Source: CAD feature listing. Evaluate the final solid. Frame: model axes, mm. A direction names the side the tool comes from. Give positions to 0.01 mm unless a question says otherwise; leave off trailing zeros. Loops run counter-clockwise (first coordinate to the right, second up) from the corner with the lowest first, then second, coordinate; pieces in that order, holes last. Notation, with made-up numbers: (74.5, 15) -> (127.5, 15) arc R21 ccw to (127.5, 47) -> close; hole circle Ø2 at (17, 20.25). An arc over 180 degrees is marked (long way). Return JSON: item names as keys, results as strings. Group by question number.
```python
from build123d import *
from build123d.topology import SkipClean

# Parameters (mm, degrees)
SKETCH7_R                  = 38.1
SKETCH7_R_2                = 18.1229
BOSS_EXTRUDE3_DEPTH        = 9.525
CUT_EXTRUDE4_REACH         = 1065.597
CUT_EXTRUDE4_END_RADIUS    = 31.75
CIRPATTERN1_COUNT          = 6
SKETCH19_R                 = 38.1
BOSS_EXTRUDE4_DEPTH        = 15.875
F_10_32_TAPPED_HOLE1_D     = 4.0386
F_10_32_TAPPED_HOLE1_DEPTH = 12.7
F_10_32_TAPPED_HOLE1_TIP   = 1.213317848


with BuildPart() as part:
    # Sketch1 → Revolve1 (revolve)
    with BuildSketch(Plane.XY, mode=Mode.PRIVATE) as revolve1_sk:
        Polygon((104.775, 1038.225), (104.775, 1044.575), (114.3, 1044.575), (114.3, 1054.1), (120.65, 1054.1), (120.65, 1044.575), (133.582417551, 1044.575), (133.582417551, 1038.225), align=None)
    revolve(revolve1_sk.sketch.rotate(Axis((184.382417551, 1006.475, 0), (-1, 0, 0)), 90), axis=Axis((184.382417551, 1006.475, 0), (-1, 0, 0)))

    # Sketch7 → Boss-Extrude3 (add)
    with BuildSketch(Plane(origin=(133.582417551, 0, 0), x_dir=(0, 0, -1), z_dir=(1, 0, 0))):
        with Locations((0, 1006.475)):
            Circle(SKETCH7_R)
        with Locations((0, 1006.475)):
            Circle(SKETCH7_R_2, mode=Mode.SUBTRACT)
    extrude(amount=-BOSS_EXTRUDE3_DEPTH)

    # Cut-Extrude4: up to this cylinder (the profile starts inside it)
    cut_extrude4_end = Plane(origin=(128.8199175, 1006.475, 0), z_dir=(1, 0, 0)) * Cylinder(CUT_EXTRUDE4_END_RADIUS, 2204.478263, mode=Mode.PRIVATE)
    # Sketch8 → Cut-Extrude4 (cut, up to the surface)
    with BuildSketch(Plane.XY, mode=Mode.PRIVATE) as cut_extrude4_sk1:
        Polygon((133.582417551, 1000.125), (133.582417551, 1012.825), (132.471311524, 1000.125), align=None)
    cut_extrude4_tool1 = extrude(cut_extrude4_sk1.sketch, amount=-CUT_EXTRUDE4_REACH, mode=Mode.PRIVATE) & cut_extrude4_end
    # Sketch8 → Cut-Extrude4 (cut, up to the surface)
    with BuildSketch(Plane.XY, mode=Mode.PRIVATE) as cut_extrude4_sk2:
        Polygon((124.057417551, 1012.825), (124.057417551, 1000.125), (125.168523578, 1012.825), align=None)
    cut_extrude4_tool2 = extrude(cut_extrude4_sk2.sketch, amount=-CUT_EXTRUDE4_REACH, mode=Mode.PRIVATE) & cut_extrude4_end
    cut_extrude4 = cut_extrude4_tool1.solids().sort_by_distance((133.212049, 1004.358333, 0))[0] + cut_extrude4_tool2.solids().sort_by_distance((124.427786, 1008.591667, 0))[0]
    add(cut_extrude4, mode=Mode.SUBTRACT)

    # Sketch18 → #10-24 Tapped Hole2 (revolve, cut)
    with BuildSketch(Plane(origin=(133.031084587, 1006.523235384, -22.225), x_dir=(0.08715574274765736, 0.9961946980917457, 0), z_dir=(0, 0, 1))):
        Polygon((0, 0), (0, 16.126824014), (1.89865, 14.986), (1.89865, 0), align=None)
    f_10_24_tapped_hole2 = revolve(axis=Axis((139.35692092, 1005.969796418, -22.225), (-0.9961946980917457, 0.08715574274765729, 0)), mode=Mode.SUBTRACT)

    # CirPattern1: Cut-Extrude4, #10-24 Tapped Hole2 ×6 about axis
    with SkipClean():  # the faces are left unmerged after this step: merging them gives an invalid solid
        cirpattern1_axis = Axis((0, 1006.475, 0), (1, 0, 0))
        add([cut_extrude4.rotate(cirpattern1_axis, i * 360 / CIRPATTERN1_COUNT) for i in range(1, CIRPATTERN1_COUNT)], mode=Mode.SUBTRACT)
        add([f_10_24_tapped_hole2.rotate(cirpattern1_axis, i * 360 / CIRPATTERN1_COUNT) for i in range(1, CIRPATTERN1_COUNT)], mode=Mode.SUBTRACT)
    add(part.part.scale(1), mode=Mode.REPLACE)  # the faces are merged on a copy

    # Sketch19 → Boss-Extrude4 (add)
    with SkipClean():  # the faces are left unmerged after this step: merging them gives an invalid solid
        with BuildSketch(Plane.ZY.offset(-120.65)):
            with BuildLine():
                Line((-47.625, 1006.475), (-47.625, 1057.275))
                Line((-47.625, 1057.275), (47.625, 1057.275))
                Line((47.625, 1057.275), (47.625, 1006.475))
                ThreePointArc((47.625, 1006.475), (0, 958.85), (-47.625, 1006.475))
            make_face()
            with Locations(Location((0, 1006.475, 0), (0, 0, 180))):
                Circle(SKETCH19_R, mode=Mode.SUBTRACT)
        extrude(amount=BOSS_EXTRUDE4_DEPTH)

    # #10-32 Tapped Hole1
    with Locations(Plane(origin=(0, 1057.275, 0), x_dir=(1, 0, 0), z_dir=(0, 1, 0))):
        with Locations((112.7125, 38.1), (112.7125, 0), (112.7125, -38.1)):
            Hole(F_10_32_TAPPED_HOLE1_D / 2, depth=F_10_32_TAPPED_HOLE1_DEPTH)
            with Locations((0, 0, -(F_10_32_TAPPED_HOLE1_DEPTH + F_10_32_TAPPED_HOLE1_TIP / 2))):  # 118° drill point
                Cone(0, F_10_32_TAPPED_HOLE1_D / 2, F_10_32_TAPPED_HOLE1_TIP, mode=Mode.SUBTRACT)


solid = part.part
```
1) Mould query, pull axis Y, two halves, no side actions, for faces 4 (the face through (113, 1032, -47.625)), 5 (the face through (133.158, 1034.695, 14.55)), 6 (the face through (112.362, 1043.572, -38.115)). Classes: released by +Y, released by -Y, zero draft, split by the parting line, or undercut.
2) Cut plane B-B on x = 107. Return loops of the section in (y, z) (3 decimals).
3) Cut plane C-C on z = 25.5. Return loops of the section in (x, y) (3 decimals), then the cut area to 3 significant figures.
4) Material intervals for line 1 (X direction, y = 1052.5, z = 38.1) (3 decimals); line 2 (X direction, y = 1029, z = 43.5) (3 decimals); line 3 (Z direction, x = 113.5, y = 1027) (3 decimals), sorted ascending.
5) Reachability of faces 1 (the face through (124.605, 985.511, 12.206)), 2 (the face through (133.16, 1033.19, -17.16)), 3 (the face through (133.582, 997, -16)) from +Z, -Z, +X, -X, +Y, -Y: full face, straight path, thin tool, end or side. Return the list, or none.
6) Contact query for flat-ended pins moving along their axis: P1, Ø4.5, axis at x = 112.71, z = 0, coming from the -Y side; P2, Ø1.5, axis at y = 1010, z = 27, coming from the -X side; P3, Ø4, axis at y = 1007.5, z = -26, coming from the -X side. Output: stop coordinate, or through.
Calculated:
{
 "1": {"face 4": "zero draft", "face 5": "undercut", "face 6": "released by +Y"},
 "2": {"outline": "(1006.475, -47.625) -> (1057.275, -47.625) -> (1057.275, 47.625) -> (1006.475, 47.625) arc R47.625 ccw to start; hole circle Ø63.5 at (1006.475, 0)"},
 "3": {"outline": "(104.775, 966.252) -> (120.65, 966.252) -> (120.65, 978.167) -> (133.582, 978.167) -> (133.582, 1000.125) -> (132.471, 1012.825) -> (133.582, 1012.825) -> (133.582, 1034.783) -> (120.65, 1034.783) -> (120.65, 1057.275) -> (104.775, 1057.275) -> (104.775, 1025.391) -> (124.057, 1025.391) -> (124.057, 1012.825) -> (125.169, 1000.125) -> (124.057, 1000.125) -> (124.057, 987.559) -> (104.775, 987.559) -> close", "area": "1,430 mm2"},
 "4": {"line 1": "104.775 to 110.693, 114.732 to 120.65", "line 2": "104.775 to 120.65", "line 3": "-47.625 to -24.224, 24.224 to 47.625"},
 "5": {"face 1": "-X", "face 2": "+X", "face 3": "+Z, -Z, +X, +Y, -Y"},
 "6": {"P1": "y = 958.85", "P2": "x = 124.24", "P3": "x = 124.53"}
}
